```python
from build123d import *

# Parameters (mm, degrees)
F0_W            = 40.5
F0_H            = 40.5
F1_DEPTH        = 2.5
F3_DEPTH        = 8.65
F4_DEPTH        = 8.65
F4_COPIES_COUNT = 4
F5_R            = 19.15
F6_DEPTH        = 11.151
F8_D            = 3.3
F8_CBORE_D      = 6.1
F8_CBORE_DEPTH  = 3


# Not quite as in the source:
# - a pattern or mirror of a feature is missing from the dataset's text; its kind, count and spacing are read off the source's solid


with BuildPart() as f1:
    # F0 (on Front) → F1 (new body)
    with BuildSketch(Plane.XZ):
        with Locations((20.25, 20.25)):
            Rectangle(F0_W, F0_H)
    extrude(amount=F1_DEPTH)

    # F2 (on face) → F3 (join)
    with BuildSketch(Plane.XZ.offset(2.5)):
        with BuildLine():
            ThreePointArc((20.25, 0), (34.568912319, 5.931087681), (40.5, 20.25))
            ThreePointArc((40.5, 20.25), (39.6168263322, 26.1651109727), (37.0443419437, 31.5642643895))
            ThreePointArc((37.0443419437, 31.5642643895), (34.568912319, 34.568912319), (31.5642643895, 37.0443419437))
            ThreePointArc((31.5642643895, 37.0443419437), (26.1651109727, 39.6168263322), (20.25, 40.5))
            ThreePointArc((20.25, 40.5), (5.931087681, 34.568912319), (0, 20.25))
            ThreePointArc((0, 20.25), (5.931087681, 5.931087681), (20.25, 0))
        make_face()
    extrude(amount=F3_DEPTH)

    # F2 (on face) → F4 (join, through all)
    with BuildSketch(Plane.XZ.offset(2.5)):
        with BuildLine():
            ThreePointArc((31.5642643895, 37.0443419437), (34.568912319, 34.568912319), (37.0443419437, 31.5642643895))
            Line((37.0443419437, 31.5642643895), (40.5, 35.0199224458))
            Line((40.5, 35.0199224458), (40.5, 40.5))
            Line((40.5, 40.5), (35.0199224458, 40.5))
            Line((35.0199224458, 40.5), (31.5642643895, 37.0443419437))
        make_face()
    f4 = extrude(amount=F4_DEPTH)

    # F4_copies: F4 ×4 about axis
    f4_copies_axis = Axis((20.25, 0, 20.25), (0, 1, 0))
    for i in range(1, F4_COPIES_COUNT):
        add(f4.rotate(f4_copies_axis, i * 360 / F4_COPIES_COUNT))

    # F5 (on face) → F6 (cut, through all)
    with BuildSketch(Plane.XZ.offset(11.15)):
        with Locations((20.25, 20.25)):
            Circle(F5_R)
    extrude(amount=-F6_DEPTH, mode=Mode.SUBTRACT)

    # F8 (through all)
    with Locations(Plane.XZ.offset(11.15)):
        with Locations((36, 36)):
            CounterBoreHole(F8_D / 2, F8_CBORE_D / 2, F8_CBORE_DEPTH)


solid = f1.part
```
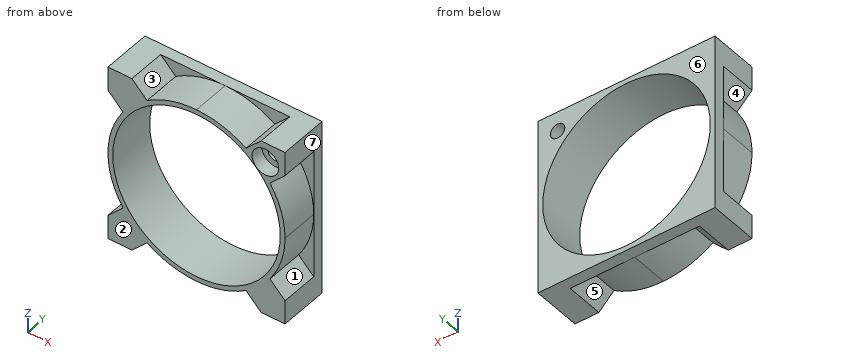
For this review, take the finished solid that the model builds, in its own axes (mm). Face numbers are marked on the shaded views. A direction names the side the tool comes from. Round coordinates to 2 decimals unless told otherwise and drop trailing zeros. Order: outer loops, then holes, each group sorted by start corner. A loop starts at its lowest first (then second) coordinate and runs counter-clockwise, first axis right, second up.
Q1. We need section B-B, the plane x = 31. Give the boundary of the cut face in (y, z).
Findings below:
outline: (-11.15, 3.09) - (-2.5, 3.09) - (-2.5, 0) - (0, 0) - (0, 4.4) - (-11.15, 4.4) - close; (-11.15, 36.1) - (0, 36.1) - (0, 40.5) - (-2.5, 40.5) - (-2.5, 37.41) - (-11.15, 37.41) - close
Q2. We need section D-D, the plane z = 36. Give the boundary of the cut face in (x, y), plus the area to 3 significant figures.
Findings below:
outline: (0, -11.15) - (9.36, -11.15) - (9.36, 0) - (0, 0) - close; (31.14, -11.15) - (32.95, -11.15) - (32.95, -8.15) - (34.35, -8.15) - (34.35, 0) - (31.14, 0) - close; (37.65, -8.15) - (39.05, -8.15) - (39.05, -11.15) - (40.5, -11.15) - (40.5, 0) - (37.65, 0) - close
area: 163 mm2
Q3. Machinability: for the marked faces 1, 2 and 3, which of the approach directions +Z, -Z, +X, -X, +Y, -Y give a long, thin tool a straight path to every point of the face, cutting with its end or side? Answer none if there is none.
Findings below:
face 1: +X, -Y
face 2: +Z, -Z, +X, -X, -Y
face 3: +Z, -Y
Q4. We need section A-A, the plane y = -9. Give the boundary of the cut face in (x, z), plus the area to 3 significant figures.
Findings below:
outline: (0, 0) - (5.48, 0) - (8.94, 3.46) arc R20.25 ccw to (31.56, 3.46) - (35.02, 0) - (40.5, 0) - (40.5, 5.48) - (37.04, 8.94) arc R20.25 ccw to (37.04, 31.56) - (40.5, 35.02) - (40.5, 40.5) - (35.02, 40.5) - (31.56, 37.04) arc R20.25 ccw to (8.94, 37.04) - (5.48, 40.5) - (0, 40.5) - (0, 35.02) - (3.46, 31.56) arc R20.25 ccw to (3.46, 8.94) - (0, 5.48) - close; hole circle Ø38.3 at (20.25, 20.25); hole circle Ø6.1 at (36, 36)
area: 311 mm2
Q5. Mouldability with a two-part tool opening along X and no side actions: class the marked faces 4, 5, 6 and 7 as pulls with the +X half, pulls with the -X half, needs draft (parallel to the pull), parting line crosses it, or undercut.
Findings below:
face 4: pulls with the -X half
face 5: undercut
face 6: needs draft
face 7: pulls with the +X half
Q6. Insertion check: P1, Ø2, axis at x = 11, y = -4.5, coming from the -Z side; P2, Ø1.7, axis at x = 31, z = 1.5, coming from the -Y side; P3, Ø1.8, axis at x = 37, z = 35, coming from the -Y side. Each pin has a flat end and moves straight along its axis. Give the tip position at first contact, or say it passes through.
Findings below:
P1: stops at z = 1.76
P2: stops at y = -2.5
P3: stops at y = -8.15
Q7. We need section C-C, the plane z = 5. Give the boundary of the cut face in (x, y).
Findings below:
outline: (0, -11.15) - (8.67, -11.15) - (8.67, 0) - (0, 0) - close; (31.83, -11.15) - (40.5, -11.15) - (40.5, 0) - (31.83, 0) - close
Q8. Wall thickness on line 1 (Z direction, x = 20.25, y = -3.75); line 2 (Z direction, x = 36, y = -9.55); line 3 (X direction, y = -6.75, z = 37.5): over which ranges is each line inside the solid? List them lowest first.
Findings below:
line 1: z = 0 to 1.1, 39.4 to 40.5
line 2: z = 0 to 9.36, 31.14 to 32.95, 39.05 to 40.5
line 3: x = 0 to 8.48, 9.64 to 11.93, 28.57 to 30.86, 32.02 to 35.31, 36.69 to 40.5
